from build123d import *

# Parameters (mm, degrees)
EXTRUDE_1_DEPTH    = 5
HOLE_WIZARD_M3_1_D = 3.2


with BuildPart() as part:
    # 草图1 → 拉伸-薄壁1 (new, symmetric)
    with BuildSketch(Plane(origin=(0, 0, 0), x_dir=(0, 0, -1), z_dir=(1, 0, 0))):
        with BuildLine():
            Line((0, 0), (0, 6))
            ThreePointArc((0, 6), (1.171572875, 8.828427125), (4, 10))
            Line((4, 10), (10, 10))
            Line((10, 10), (10, 8))
            Line((10, 8), (4, 8))
            ThreePointArc((4, 8), (2.585786438, 7.414213562), (2, 6))
            Line((2, 6), (2, 0))
            Line((2, 0), (0, 0))
        make_face()
    extrude(amount=EXTRUDE_1_DEPTH, both=True)

    # M3 间隙孔1 (through all)
    with Locations(Plane(origin=(0, 10, 0), x_dir=(1, 0, 0), z_dir=(0, 1, 0))):
        with Locations((0, 7)):
            Hole(HOLE_WIZARD_M3_1_D / 2)


solid = part.part
Part model, mm, in its own coordinate system. A direction names the side the tool comes from. Give positions to 0.01 mm unless a question says otherwise; leave off trailing zeros. Loops run counter-clockwise (first coordinate to the right, second up) from the corner with the lowest first, then second, coordinate; pieces in that order, holes last.
(1) Band-saw the part on C-C (x = -4). Write the cut outline in (y, z), and give its area (3 significant figures).
Return value:
outline: (0, -2) - (6, -2) arc R2 cw to (8, -4) - (8, -10) - (10, -10) - (10, -4) arc R4 ccw to (6, 0) - (0, 0) - close
area: 33.4 mm2
(2) 3-axis set-ups, long thin cutter, end or side, ignore diameter. For faces 5 (the flat face through (0, 3, -2)), 6 (the flat face through (0, 9, -10)): which of +Z, -Z, +X, -X, +Y, -Y reach the whole face in a straight line?
Return value:
face 5: -Z, +X, -X, -Y
face 6: -Z, +X, -X, +Y, -Y
(3) Pin check, flat tips, straight feed: pin 1 (5 mm diameter, centred on x = -1, y = 3.5, fed in from -Z); pin 2 (3 mm diameter, centred on x = -2, y = 7.5, fed in from -Z); pin 3 (3 mm diameter, centred on x = 0, z = -7, fed in from -Y); pin 4 (4 mm diameter, centred on x = 1.5, z = -7, fed in from -Y). Stop position of each tip, or through.
Return value:
pin 1: stops at z = -2
pin 2: stops at z = -10
pin 3: passes through
pin 4: stops at y = 8
(4) Band-saw the part on D-D (y = 5.5). Write the cut outline in (x, z), and give its area (3 significant figures).
Return value:
outline: (-5, -2) - (5, -2) - (5, 0) - (-5, 0) - close
area: 20.0 mm2
(5) Band-saw the part on A-A (z = -7). Write the cut outline in (x, y).
Return value:
outline: (-5, 8) - (-1.6, 8) - (-1.6, 10) - (-5, 10) - close; (1.6, 8) - (5, 8) - (5, 10) - (1.6, 10) - close
(6) Band-saw the part on B-B (x = 0). Write the cut outline in (y, z), and give its area (3 significant figures).
Return value:
outline: (0, -2) - (6, -2) arc R2 cw to (8, -4) - (8, -5.4) - (10, -5.4) - (10, -4) arc R4 ccw to (6, 0) - (0, 0) - close; (8, -10) - (10, -10) - (10, -8.6) - (8, -8.6) - close
area: 27.0 mm2
(7) Pull direction X, two halves, no side cores. Call faces 1 (the cylindrical face through (0.35, 8.99, -5.44)), 2 (the flat face through (5, 8, -3)), 3 (the flat face through (-5, 8, -3)), 4 (the flat face through (1.2, 8, -5.7)): pulls with the +X half, pulls with the -X half, needs draft (parallel to the pull), parting line crosses it, or undercut.
Return value:
face 1: undercut
face 2: pulls with the +X half
face 3: pulls with the -X half
face 4: needs draft
(8) Drill centre lines: line 1 along X through (y, z) = (9.3, -7); line 2 along Y through (x, z) = (0, -4.5); line 3 along Z through (x, y) = (3.75, 5). Where is each one in solid material? Low to high.
Return value:
line 1: x = -5 to -1.6, 1.6 to 5
line 2: y = 8 to 10
line 3: z = -2 to 0
